Here's how the part is built. I have some questions about the finished solid (model axes, mm). A direction names the side the tool comes from. Coordinates: 2 decimals unless noted, no trailing zeros. Loops run counter-clockwise (first coordinate to the right, second up) from the corner with the lowest first, then second, coordinate; pieces in that order, holes last. Notation, with made-up numbers: (-32, -15.75) -> (26, -15.75) arc R18 cw to (26, -4.75) -> close; hole circle Ø6 at (38.25, 36.5). An arc over 180 degrees is marked (long way). Answer as a JSON object with one key per item and string values. Group by question number.
1) I want a section at A-A (z = 24.25). Write out the boundary of the cut face in (x, y), then the cut area to 3 significant figures.
2) I'm going to push flat-ended pins straight in: pin 1 (1.5 mm diameter, centred on y = -61.5, z = 23.5, fed in from +X); pin 2 (3 mm diameter, centred on x = -17, z = 22, fed in from -Y); pin 3 (1.5 mm diameter, centred on y = -62, z = 21.5, fed in from -X). Where does each tip first touch, or does it pass through?
3) I want a section at B-B (x = -15). Write out the boundary of the cut face in (y, z).
4) Which directions (+Z, -Z, +X, -X, +Y, -Y) give clear straight access to the entire face, cutting with the end or side of a thin tool? Please do faces 4 (the flat face through (-16, -58.45, 22)), 5 (the flat face through (-7, -3, 25.898)).
5) I need wall thicknesses on probe 1 along Y at (x, z) = (0.5, 23). Which ranges of the line are inside material? Lowest first, please. Write a range as [from, to].
6) If we mould it in two halves opening along Y, with no side actions, what happens to faces 1 (the flat face through (-7, 58.45, 22)), 2 (the flat face through (0.39, -61, 22)), 3 (the flat face through (3, -58.45, 22))? For each: +Y half, -Y half, draft (parallel to the pull), parting line (faces both ways), or undercut.
```python
from build123d import *

# Parameters (mm, degrees)
F0_W     = 25.2
F0_H     = 7.2
F1_DEPTH = 58.45
F2_W     = 13.700049
F2_H     = 7.2
F3_DEPTH = 5


with BuildPart() as f1:
    # F0 (on Front) → F1 (new body, symmetric)
    with BuildSketch(Plane.XZ):
        with Locations((-6.539625, 22.297869)):
            Rectangle(F0_W, F0_H)
    extrude(amount=F1_DEPTH, both=True)

    # F2 (on face) → F3 (join)
    with BuildSketch(Plane.XZ.offset(58.45)):
        with Locations((-6.460382, 22.297869)):
            Rectangle(F2_W, F2_H)
    extrude(amount=F3_DEPTH)


solid = f1.part
```
Determined:
{
 "1": {"outline": "(-19.14, -58.45) -> (-13.31, -58.45) -> (-13.31, -63.45) -> (0.39, -63.45) -> (0.39, -58.45) -> (6.06, -58.45) -> (6.06, 58.45) -> (-19.14, 58.45) -> close", "area": "3,010 mm^2"},
 "2": {"pin 1": "x = 0.39", "pin 2": "y = -58.45", "pin 3": "x = -13.31"},
 "3": {"outline": "(-58.45, 18.7) -> (58.45, 18.7) -> (58.45, 25.9) -> (-58.45, 25.9) -> close"},
 "4": {"face 4": "+Z, -Z, -X, -Y", "face 5": "+Z, +X, -X, +Y, -Y"},
 "5": {"probe 1": "[-58.45, 58.45]"},
 "6": {"face 1": "+Y half", "face 2": "draft", "face 3": "-Y half"}
}
